Work out the finished part from the listing and answer in its coordinate system (mm). Round coordinates to 2 decimals unless told otherwise and drop trailing zeros. Write each loop counter-clockwise with the first axis right and the second up, starting at its lowest first coordinate (ties: lowest second). Pieces come first, ordered by that corner, then holes. Notation, with made-up numbers: (25.5, -37.5) - (75.5, -37.5) arc R25 ccw to (75.5, -24.5) - close; hole circle Ø10 at (-15, -23). An arc over 180 degrees is marked (long way). Answer as a JSON object with one key per item and string values.
```python
from build123d import *

# Parameters (mm, degrees)
CROQUIS1_W              = 1000
CROQUIS1_H              = 1000
SALIENTE_EXTRUIR1_DEPTH = 350
CHAFL_N1_SIZE           = 180
CHAFL_N1_SIZE2          = 311.769145362
CROQUIS2_W              = 75
CROQUIS2_H              = 75
SALIENTE_EXTRUIR2_DEPTH = 20


with BuildPart() as part:
    # Croquis1 → Saliente-Extruir1 (new body)
    with BuildSketch(Plane(origin=(0, 0, 0), x_dir=(1, 0, 0), z_dir=(0, 1, 0))):
        Rectangle(CROQUIS1_W, CROQUIS1_H)
    extrude(amount=SALIENTE_EXTRUIR1_DEPTH)

    # Chaflán1
    chafl_n1_edges = [part.edges().sort_by_distance(p)[0] for p in [
        (0, 0, -500),
        (500, 0, 0),
        (0, 0, 500),
        (-500, 0, 0),
    ]]
    chafl_n1_side = [part.faces().sort_by_distance(p)[0] for p in [
        (0, 0, 0),
    ]]
    chamfer(chafl_n1_edges, length=CHAFL_N1_SIZE, length2=CHAFL_N1_SIZE2, reference=chafl_n1_side[0])

    # Croquis2 → Saliente-Extruir2 (add)
    with BuildSketch(Plane.XZ):
        with Locations((-282.5, 282.5)):
            Rectangle(CROQUIS2_W, CROQUIS2_H)
        with Locations((282.5, 282.5)):
            Rectangle(CROQUIS2_W, CROQUIS2_H)
        with Locations((282.5, -282.5)):
            Rectangle(CROQUIS2_W, CROQUIS2_H)
        with Locations((-282.5, -282.5)):
            Rectangle(CROQUIS2_W, CROQUIS2_H)
    extrude(amount=SALIENTE_EXTRUIR2_DEPTH)


solid = part.part
```
Item 1: Each of these flat-tipped pins is pushed along its axis until it touches: P1, Ø10, axis at x = 291.5, y = -10, coming from the +Z side; P2, Ø16, axis at x = 269.5, y = -11, coming from the -Z side; P3, Ø22, axis at y = -13, z = -299, coming from the +X side. Where does it stop, or does it pass through?
Results found:
{"P1": "z = 320", "P2": "z = -320", "P3": "x = 320"}
Item 2: A cutting plane is placed at B-B (x = -398). Write down the section's boundary in (y, z), and give its area (3 significant figures).
Results found:
{"outline": "(135.1, -398) - (311.77, -500) - (350, -500) - (350, 500) - (311.77, 500) - (135.1, 398) - close", "area": "197,000 mm²"}
Item 3: A cutting plane is placed at D-D (y = 89). Write down the section's boundary in (x, z).
Results found:
{"outline": "(-371.38, -371.38) - (371.38, -371.38) - (371.38, 371.38) - (-371.38, 371.38) - close"}
Item 4: A cutting plane is placed at C-C (y = 30.5). Write down the section's boundary in (x, z), and give its area (3 significant figures).
Results found:
{"outline": "(-337.61, -337.61) - (337.61, -337.61) - (337.61, 337.61) - (-337.61, 337.61) - close", "area": "456,000 mm²"}
Item 5: Consider line 1 along Y through (x, z) = (-173.5, 303.5); line 2 along X through (y, z) = (229, -71.5); line 3 along Y through (x, z) = (-327.5, 299). Determine where each line is inside the solid, lowest interval first.
Results found:
{"line 1": "0 to 350", "line 2": "-452.21 to 452.21", "line 3": "12.99 to 350"}
Item 6: A cutting plane is placed at A-A (z = -203.5). Write down the section's boundary in (x, y).
Results found:
{"outline": "(-500, 311.77) - (-320, 0) - (320, 0) - (500, 311.77) - (500, 350) - (-500, 350) - close"}
Item 7: Determine the mould class of faces 1 (the flat face through (-500, 331, 7)), 2 (the flat face through (-4, 0, -4)), 3 (the flat face through (-7, 158.07, -411.26)) for opening direction Z: pulls with the +Z half, pulls with the -Z half, needs draft (parallel to the pull), parting line crosses it, or undercut.
Results found:
{"face 1": "needs draft", "face 2": "undercut", "face 3": "pulls with the -Z half"}
